The listing builds one solid part. Answer for the finished solid, in the listing's coordinates (mm). Round coordinates to 2 decimals unless told otherwise and drop trailing zeros. Order: outer loops, then holes, each group sorted by start corner. A loop starts at its lowest first (then second) coordinate and runs counter-clockwise, first axis right, second up. Notation, with made-up numbers: (-14, -10.75) -> (28, -10.75) arc R18 cw to (28, 11.25) -> close; hole circle Ø3 at (72.5, -23.5). An arc over 180 degrees is marked (long way). Return JSON: item names as keys, results as strings. Group by question number.
(1) The part is cut by section A-A (x = 54.5). Determine the outline of the cut face in (y, z), plus the area to 3 significant figures.
(2) Consider line 1 (X direction, y = -23, z = 1); line 2 (X direction, y = -6, z = 2.35); line 3 (X direction, y = 5, z = 1.95). Determine where each line is inside the solid, lowest interval first. Write a range as [from, to].
(3) The part is cut by section B-B (z = 1.55). Count the separate pieces of the cut face and the enclosed holes in it, plus the area to 3 significant figures.
(4) Each of these flat-tipped pins is pushed along its axis until it touches: pin 1 (3 mm diameter, centred on x = 39, y = 8.5, fed in from -Z); pin 2 (1.2 mm diameter, centred on x = 55, z = 1.5, fed in from +Y). Where does it stop, or does it pass through?
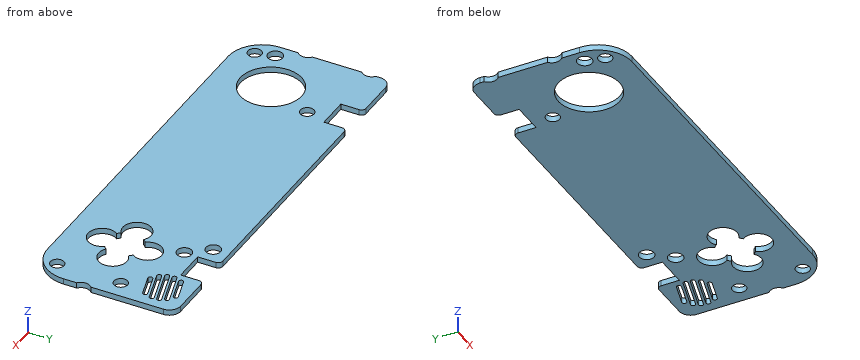
from build123d import *

# Parameters (mm, degrees)
BOSS_EXTRU_1_DEPTH       = 2.5
JOYSTICK_R               = 13.5
ENL_V_MAT_EXTRU_2_DEPTH  = 2.5
ESQUISSE2_W              = 14
ESQUISSE2_H              = 10
ENL_V_MAT_EXTRU_3_DEPTH  = 10
CONG_1_R                 = 2
CONG_2_R                 = 2
ESQUISSE3_W              = 14
ESQUISSE3_H              = 10
ENL_V_MAT_EXTRU_4_DEPTH  = 10
CONG_3_R                 = 2
CONG_4_R                 = 2
F_12X12_BUTTON_R         = 6.2
ENL_V_MAT_EXTRU_5_DEPTH  = 10
ENL_V_MAT_EXTRU_8_DEPTH  = 10
ESQUISSE5_R              = 3
ESQUISSE5_R_2            = 3.25
ENL_V_MAT_EXTRU_9_DEPTH  = 10
ESQUISSE6_R              = 4
ENL_V_MAT_EXTRU_11_DEPTH = 10


with BuildPart() as part:
    # Esquisse1 → Boss.-Extru.1 (new body)
    with BuildSketch(Plane.XY):
        with BuildLine():
            Line((-89.203921136, 33.34478673), (79.796078864, 33.34478673))
            ThreePointArc((79.796078864, 33.34478673), (83.33161277, 31.880320636), (84.796078864, 28.34478673))
            Line((84.796078864, 28.34478673), (84.796078864, -15.65521327))
            ThreePointArc((84.796078864, -15.65521327), (80.402680581, -26.261814988), (69.796078864, -30.65521327))
            Line((69.796078864, -30.65521327), (-79.203921136, -30.65521327))
            ThreePointArc((-79.203921136, -30.65521327), (-89.810522854, -26.261814988), (-94.203921136, -15.65521327))
            Line((-94.203921136, -15.65521327), (-94.203921136, 28.34478673))
            ThreePointArc((-94.203921136, 28.34478673), (-92.739455042, 31.880320636), (-89.203921136, 33.34478673))
        make_face()
    extrude(amount=BOSS_EXTRU_1_DEPTH)

    # Joystick → Enlèv. mat.-Extru.2 (cut)
    with BuildSketch(Plane.XY.offset(2.5)):
        with Locations((-68.703921136, -6.15521327)):
            Circle(JOYSTICK_R)
    extrude(amount=-ENL_V_MAT_EXTRU_2_DEPTH, mode=Mode.SUBTRACT)

    # Esquisse2 → Enlèv. mat.-Extru.3 (cut)
    with BuildSketch(Plane.XY.offset(2.5)):
        with Locations((54.066078864, 28.34478673)):
            Rectangle(ESQUISSE2_W, ESQUISSE2_H)
    extrude(amount=-ENL_V_MAT_EXTRU_3_DEPTH, mode=Mode.SUBTRACT)

    # Congé1
    cong_1_edges = [part.edges().sort_by_distance(p)[0] for p in [
        (47.066078864, 33.34478673, 1.25),
    ]]
    fillet(cong_1_edges, radius=CONG_1_R)

    # Congé2
    cong_2_edges = [part.edges().sort_by_distance(p)[0] for p in [
        (61.066078864, 33.34478673, 1.25),
    ]]
    fillet(cong_2_edges, radius=CONG_2_R)

    # Esquisse3 → Enlèv. mat.-Extru.4 (cut)
    with BuildSketch(Plane.XY.offset(2.5)):
        with Locations((-64.113921136, 28.34478673)):
            Rectangle(ESQUISSE3_W, ESQUISSE3_H)
    extrude(amount=-ENL_V_MAT_EXTRU_4_DEPTH, mode=Mode.SUBTRACT)

    # Congé3
    cong_3_edges = [part.edges().sort_by_distance(p)[0] for p in [
        (-71.113921136, 33.34478673, 1.25),
    ]]
    fillet(cong_3_edges, radius=CONG_3_R)

    # Congé4
    cong_4_edges = [part.edges().sort_by_distance(p)[0] for p in [
        (-57.113921136, 33.34478673, 1.25),
    ]]
    fillet(cong_4_edges, radius=CONG_4_R)

    # 12x12 Button → Enlèv. mat.-Extru.5 (cut)
    with BuildSketch(Plane.XY.offset(2.5)):
        with BuildLine():
            ThreePointArc((46.518078864, -0.6967139), (48.342086437, -2.883607238), (48.996078864, -5.65521327))
            ThreePointArc((48.996078864, -5.65521327), (48.342086437, -8.426819303), (46.518078864, -10.61371264))
            ThreePointArc((46.518078864, -10.61371264), (47.139224614, -11.31206752), (47.837579494, -11.93321327))
            ThreePointArc((47.837579494, -11.93321327), (52.796078864, -9.45521327), (57.754578233, -11.93321327))
            ThreePointArc((57.754578233, -11.93321327), (58.452933113, -11.31206752), (59.074078864, -10.61371264))
            ThreePointArc((59.074078864, -10.61371264), (56.596078864, -5.65521327), (59.074078864, -0.6967139))
            ThreePointArc((59.074078864, -0.6967139), (58.452933113, 0.001640979), (57.754578233, 0.62278673))
            ThreePointArc((57.754578233, 0.62278673), (52.796078864, -1.85521327), (47.837579494, 0.62278673))
            ThreePointArc((47.837579494, 0.62278673), (47.139224614, 0.001640979), (46.518078864, -0.6967139))
        make_face()
        with Locations((42.796078864, -5.65521327)):
            Circle(F_12X12_BUTTON_R)
        with Locations((52.796078864, 4.34478673)):
            Circle(F_12X12_BUTTON_R)
        with Locations((62.796078864, -5.65521327)):
            Circle(F_12X12_BUTTON_R)
        with Locations((52.796078864, -15.65521327)):
            Circle(F_12X12_BUTTON_R)
    extrude(amount=-ENL_V_MAT_EXTRU_5_DEPTH, mode=Mode.SUBTRACT)

    # Esquisse4 → Enlèv. mat.-Extru.8 (cut)
    with BuildSketch(Plane.XY.offset(2.5)):
        with BuildLine():
            Line((63.848163441, 19.991775112), (79.166394029, 24.612577171))
            ThreePointArc((79.166394029, 24.612577171), (80.412583569, 23.943987888), (79.743994286, 22.697798347))
            Line((79.743994286, 22.697798347), (64.425763698, 18.076996289))
            ThreePointArc((64.425763698, 18.076996289), (63.179574158, 18.745585572), (63.848163441, 19.991775112))
        make_face()
        with BuildLine():
            Line((63.539756046, 23.02230266), (77.747509179, 27.308125004))
            ThreePointArc((77.747509179, 27.308125004), (78.993698719, 26.639535721), (78.325109436, 25.39334618))
            Line((78.325109436, 25.39334618), (64.117356303, 21.107523836))
            ThreePointArc((64.117356303, 21.107523836), (62.871166763, 21.776113119), (63.539756046, 23.02230266))
        make_face()
        with BuildLine():
            Line((64.732924902, 26.557541009), (74.798428352, 29.593838105))
            ThreePointArc((74.798428352, 29.593838105), (76.044617893, 28.925248822), (75.37602861, 27.679059282))
            Line((75.37602861, 27.679059282), (65.31052516, 24.642762185))
            ThreePointArc((65.31052516, 24.642762185), (64.064335619, 25.311351468), (64.732924902, 26.557541009))
        make_face()
        with BuildLine():
            Line((65.314724126, 17.237366416), (79.467627817, 21.506643219))
            ThreePointArc((79.467627817, 21.506643219), (80.713811222, 20.838057228), (80.04522523, 19.591873823))
            Line((80.04522523, 19.591873823), (65.89232154, 15.32259702))
            ThreePointArc((65.89232154, 15.32259702), (64.646138135, 15.991183011), (65.314724126, 17.237366416))
        make_face()
        with BuildLine():
            Line((68.322797362, 14.963301678), (78.218865725, 17.948488042))
            ThreePointArc((78.218865725, 17.948488042), (79.465055266, 17.279898759), (78.796465983, 16.033709218))
            Line((78.796465983, 16.033709218), (68.900397619, 13.048522855))
            ThreePointArc((68.900397619, 13.048522855), (67.654208079, 13.717112138), (68.322797362, 14.963301678))
        make_face()
    extrude(amount=-ENL_V_MAT_EXTRU_8_DEPTH, mode=Mode.SUBTRACT)

    # Esquisse5 → Enlèv. mat.-Extru.9 (cut)
    with BuildSketch(Plane.XY.offset(2.5)):
        with Locations((76.796078864, -22.65521327)):
            Circle(ESQUISSE5_R)
        with Locations((-86.203921136, -22.65521327)):
            Circle(ESQUISSE5_R)
        with Locations((76.796078864, 5.34478673)):
            Circle(ESQUISSE5_R)
        with Locations((-60.203921136, 14.34478673)):
            Circle(ESQUISSE5_R)
        with Locations((-88.203921136, -14.65521327)):
            Circle(ESQUISSE5_R_2)
        with Locations((39.796078864, 26.34478673)):
            Circle(ESQUISSE5_R_2)
        with Locations((46.796078864, 17.34478673)):
            Circle(ESQUISSE5_R_2)
    extrude(amount=-ENL_V_MAT_EXTRU_9_DEPTH, mode=Mode.SUBTRACT)

    # Esquisse6 → Enlèv. mat.-Extru.11 (cut)
    with BuildSketch(Plane.XY.offset(2.5)):
        with Locations((-96.703921136, -4.65521327)):
            Circle(ESQUISSE6_R)
        with Locations((-96.703921136, 23.34478673)):
            Circle(ESQUISSE6_R)
        with Locations((87.296078864, -6.65521327)):
            Circle(ESQUISSE6_R)
    extrude(amount=-ENL_V_MAT_EXTRU_11_DEPTH, mode=Mode.SUBTRACT)


solid = part.part
Answer below:
{
 "1": {"outline": "(-30.66, 0) -> (-21.62, 0) -> (-21.62, 2.5) -> (-30.66, 2.5) -> close; (10.31, 0) -> (23.34, 0) -> (23.34, 2.5) -> (10.31, 2.5) -> close", "area": "55.2 mm²"},
 "2": {"line 1": "x = [-92.28, -89.18], [-83.22, 73.82], [79.78, 82.87]", "line 2": "x = [-92.94, -82.2], [-55.2, 36.61], [68.99, 83.35]", "line 3": "x = [-94.2, -76.31], [-61.1, 46.63], [58.96, 73.82], [79.78, 84.8]"},
 "3": {"separate pieces": "1", "enclosed holes": "14", "area": "9,540 mm²"},
 "4": {"pin 1": "stops at z = 0", "pin 2": "stops at y = 23.34"}
}
